Print and shaded views of the part. All mm, measured from the part's lowest x, y and z. A direction names the side the tool comes from. Give positions to 0.01 mm unless a question says otherwise; leave off trailing zeros. Loops run counter-clockwise (first coordinate to the right, second up) from the corner with the lowest first, then second, coordinate; pieces in that order, holes last. Notation, with made-up numbers: M -20,38.5 L 36,38.5 A19 ccw 36,51.5 Z; hole C 19.25,-26.75 d2. An arc over 180 degrees is marked long. Put each result on its own line as item: value. Start each with the question number.
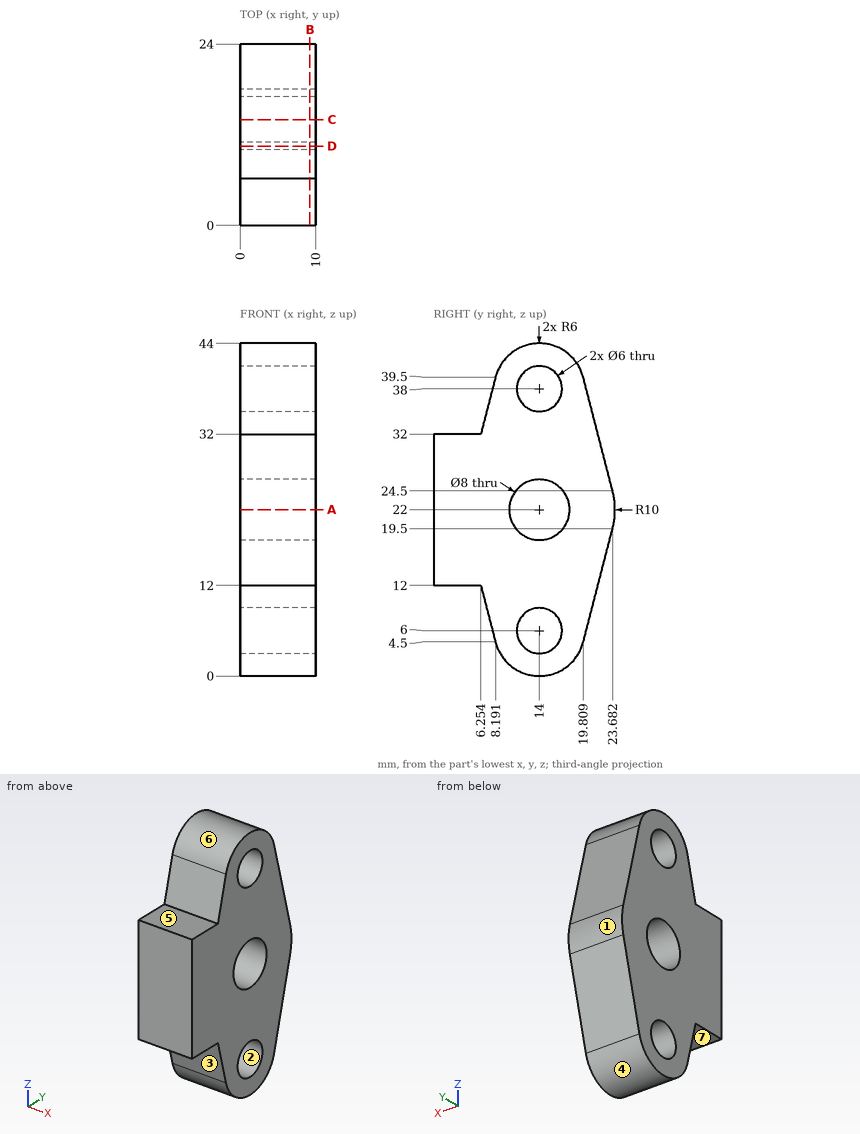
1) Pin check, flat tips, straight feed: pin 1 Ø5 at (x, y) = (2.5, 3.5) entering from +Z; pin 2 Ø4 at (y, z) = (12.5, 8.5) entering from -X; pin 3 Ø1.5 at (x, y) = (1.5, 8.5) entering from +Z (1 decimal); pin 4 Ø1.9 at (x, y) = (6, 4) entering from -Z. Stop position of each tip, or through.
2) Which spindle directions (+Z, -Z, +X, -X, +Y, -Y) get a long thin tool onto all of the face, cutting with end or side? Do the marked faces 5, 6 and 7. Say none if no direction does.
3) Wall check: L1, parallel to Y at x = 6.5, z = 22; L2, parallel to Z at x = 9.75, y = 12.75; L3, parallel to Z at x = 9.25, y = 11.5 (1 decimal). Give the ranges that are in metal, low to high.
4) Band-saw the part on C-C on y = 14. Give the cut face in (x, z), then the cut area to 3 significant figures.
5) Band-saw the part on A-A on z = 22. Give the cut face in (x, y), then the cut area to 3 significant figures.
6) Band-saw the part on B-B on x = 9.25. Give the cut face in (y, z), then the cut area to 3 significant figures.
7) Band-saw the part on D-D on y = 10.5. Give the cut face in (x, z).
8) Mould opens along Y. For the marked faces 1, 2, 3 and 4 say: +Y half, -Y half, draft (parallel to the pull), parting line (faces both ways), or undercut.
Evaluation:
1. pin 1: z = 32
1. pin 2: x = 0
1. pin 3: z = 41.7
1. pin 4: z = 12
2. face 5: +Z, +X, -X, -Y
2. face 6: +Z, +X, -X
2. face 7: -Z, +X, -X, -Y
3. L1: 0 to 10, 18 to 24
3. L2: 0.13 to 3.27, 8.73 to 18.2, 25.8 to 35.27, 40.73 to 43.87
3. L3: 0.5 to 4.3, 7.7 to 18.9, 25.1 to 36.3, 39.7 to 43.5
4. outline: M 0,0 L 10,0 L 10,3 L 0,3 Z; M 0,9 L 10,9 L 10,18 L 0,18 Z; M 0,26 L 10,26 L 10,35 L 0,35 Z; M 0,41 L 10,41 L 10,44 L 0,44 Z
4. area: 240 mm2
5. outline: M 0,0 L 10,0 L 10,10 L 0,10 Z; M 0,18 L 10,18 L 10,24 L 0,24 Z
5. area: 160 mm2
6. outline: M 0,12 L 6.25,12 L 8.19,4.5 A6 ccw 19.81,4.5 L 23.68,19.5 A10 ccw 23.68,24.5 L 19.81,39.5 A6 ccw 8.19,39.5 L 6.25,32 L 0,32 Z; hole C 14,22 d8; hole C 14,6 d6; hole C 14,38 d6
6. area: 634 mm2
7. outline: M 0,1.13 L 10,1.13 L 10,20.06 L 0,20.06 Z; M 0,23.94 L 10,23.94 L 10,42.87 L 0,42.87 Z
8. face 1: +Y half
8. face 2: undercut
8. face 3: -Y half
8. face 4: parting line
